Here's how the part is built. I have some questions about the finished solid (model axes, mm). Give positions to 0.01 mm unless a question says otherwise; leave off trailing zeros. Order: outer loops, then holes, each group sorted by start corner. A loop starts at its lowest first (then second) coordinate and runs counter-clockwise, first axis right, second up.
from build123d import *

# Parameters (mm, degrees)
SKETCH_1_R          = 6
SKETCH_1_R_2        = 5
EXTRUDE_1_DEPTH     = 10
CUT_EXTRUDE_1_DEPTH = 20


with BuildPart() as part:
    # 草图1 → 凸台-拉伸1 (new body)
    with BuildSketch(Plane.XY):
        Circle(SKETCH_1_R)
        Circle(SKETCH_1_R_2, mode=Mode.SUBTRACT)
    extrude(amount=EXTRUDE_1_DEPTH)

    # 草图2 → 切除-拉伸1 (cut)
    with BuildSketch(Plane.XY.offset(10)):
        Polygon((0, 0), (0, 6), (0.587596227, 6.386088304), align=None)
    extrude(amount=-CUT_EXTRUDE_1_DEPTH, mode=Mode.SUBTRACT)


solid = part.part
Q1. If we section it at B-B on x = -3: List the corners of the cut face in (y, z) for me, plus the area to 3 significant figures.
Filled sheet:
outline: (-5.2, 0) - (-4, 0) - (-4, 10) - (-5.2, 10) - close; (4, 0) - (5.2, 0) - (5.2, 10) - (4, 10) - close
area: 23.9 mm2
Q2. I need wall thicknesses on L1, parallel to X at y = 0, z = 6.5; L2, parallel to Y at x = 0.75, z = 4.5; L3, parallel to Y at x = 4.5, z = 2.75. Which ranges of each line are inside material? Lowest first, please.
Filled sheet:
L1: x = -6 to -5, 5 to 6
L2: y = -5.95 to -4.94, 4.94 to 5.95
L3: y = -3.97 to -2.18, 2.18 to 3.97
Q3. If we section it at A-A on y = -0.5: List the corners of the cut face in (x, z) for me, plus the area to 3 significant figures.
Filled sheet:
outline: (-5.98, 0) - (-4.97, 0) - (-4.97, 10) - (-5.98, 10) - close; (4.97, 0) - (5.98, 0) - (5.98, 10) - (4.97, 10) - close
area: 20.1 mm2
Q4. I'm going to push flat-ended pins straight in: P1, Ø1.1, axis at y = 5.5, z = 4, coming from the +X side; P2, Ø6, axis at x = -2.5, y = 1, coming from the +Z side; P3, Ø3, axis at y = -3.5, z = 1.5, coming from the -X side. Where does each tip first touch, or does it pass through?
Filled sheet:
P1: stops at x = 3.39
P2: stops at z = 10
P3: stops at x = -5.66
Q5. Thinking about a two-plate mould opening in X: for faces 1 (the face through (0.505, 5.484, 5.07)), 2 (the face through (0, 5.5, 5.1)), 3 (the face through (-2.7, -4.4, 0)), which applies, released by +X, released by -X, zero draft, split by the parting line, or undercut?
Filled sheet:
face 1: undercut
face 2: undercut
face 3: zero draft
Q6. If we section it at C-C on z = 7: List the corners of the cut face in (x, y) for me, plus the area to 3 significant figures.
Filled sheet:
outline: (0, 5) - (0, 6) arc R6 ccw (long way) to (0.55, 5.97) - (0.46, 4.98) arc R5 cw (long way) to start
area: 34.1 mm2
